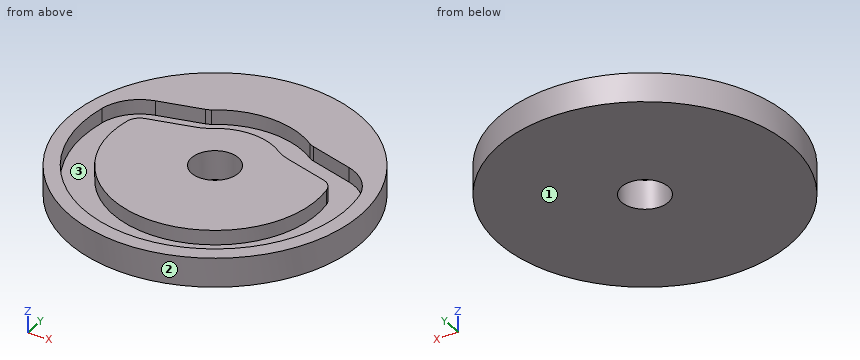
```python
from build123d import *

# Parameters (mm, degrees)
SKETCH_1_R            = 50
EXTRUDE_1_DEPTH       = 10
CUT_EXTRUDE_1_DEPTH   = 5
SKETCH_4_R            = 8
CUT_EXTRUDE_1_2_DEPTH = 72.414284285


with BuildPart() as part:
    # 草图1 → 凸台-拉伸1 (new body)
    with BuildSketch(Plane.XY):
        Circle(SKETCH_1_R)
    extrude(amount=EXTRUDE_1_DEPTH)

    # 草图2 → Cut-Extrude 1 (cut)
    with BuildSketch(Plane.XY.offset(10)):
        with BuildLine():
            ThreePointArc((44.226450487, 8.307892471), (0, -45), (-44.226450487, 8.307892471))
            ThreePointArc((-44.226450487, 8.307892471), (-40.486781839, 15.733956697), (-33.366586001, 20.027482375))
            Line((-33.366586001, 20.027482375), (-18.55842138, 23.995318126))
            ThreePointArc((-18.55842138, 23.995318126), (-17.756990045, 24.285259115), (-17.016442805, 24.70709765))
            ThreePointArc((-17.016442805, 24.70709765), (0, 30), (17.016442805, 24.70709765))
            ThreePointArc((17.016442805, 24.70709765), (17.756990045, 24.285259115), (18.55842138, 23.995318126))
            Line((18.55842138, 23.995318126), (33.366586001, 20.027482375))
            ThreePointArc((33.366586001, 20.027482375), (40.486781839, 15.733956697), (44.226450487, 8.307892471))
        make_face()
        with BuildLine():
            ThreePointArc((34.398350379, 6.461694144), (0, -35), (-34.398350379, 6.461694144))
            ThreePointArc((-34.398350379, 6.461694144), (-33.151794163, 8.937048886), (-30.77839555, 10.368224112))
            Line((-30.77839555, 10.368224112), (-15.970230929, 14.336059864))
            ThreePointArc((-15.970230929, 14.336059864), (-13.565936922, 15.20588283), (-11.344295203, 16.471398433))
            ThreePointArc((-11.344295203, 16.471398433), (0, 20), (11.344295203, 16.471398433))
            ThreePointArc((11.344295203, 16.471398433), (13.565936922, 15.20588283), (15.970230929, 14.336059864))
            Line((15.970230929, 14.336059864), (30.77839555, 10.368224112))
            ThreePointArc((30.77839555, 10.368224112), (33.151794163, 8.937048886), (34.398350379, 6.461694144))
        make_face(mode=Mode.SUBTRACT)
    extrude(amount=-CUT_EXTRUDE_1_DEPTH, mode=Mode.SUBTRACT)

    # 草图4 → Cut-Extrude 1 2 (cut, through all)
    with BuildSketch(Plane.XY.offset(10)):
        Circle(SKETCH_4_R)
    extrude(amount=-CUT_EXTRUDE_1_2_DEPTH, mode=Mode.SUBTRACT)


solid = part.part
```
Build history of the part. All positions in model axes, mm. Face numbers are marked on the shaded views. Round coordinates to 2 decimals unless told otherwise and drop trailing zeros. Write each loop counter-clockwise with the first axis right and the second up, starting at its lowest first coordinate (ties: lowest second). Pieces come first, ordered by that corner, then holes. Notation, with made-up numbers: (13.5, -4.5) -> (26.5, -4.5) arc R20 cw to (26.5, 7.5) -> close; hole circle Ø6 at (-6.75, -22). An arc over 180 degrees is marked (long way). Put each result on its own line as item: value.
Item 1: Wall check: probe 1 along Y at (x, z) = (-0.5, 8.75); probe 2 along Y at (x, z) = (19, 6); probe 3 along X at (y, z) = (-9, 6). Give the ranges that are in metal, low to high. Write a range as from..to.
Here are the results:
probe 1: y = -50..-45, -35..-7.98, 7.98..19.99, 30..50
probe 2: y = -46.25..-40.79, -29.39..13.52, 23.88..46.25
probe 3: x = -49.18..-44.09, -33.82..33.82, 44.09..49.18
Item 2: Two-plate mould, pull along Y, no slides. Class the marked faces 1, 2 and 3: pulls with the +Y half, pulls with the -Y half, needs draft (parallel to the pull), parting line crosses it, or undercut.
Here are the results:
face 1: needs draft
face 2: parting line crosses it
face 3: undercut
Item 3: Slice it at B-B, the plane x = 0. Give the cut face in (y, z), plus the area to 3 significant figures.
Here are the results:
outline: (-50, 0) -> (-8, 0) -> (-8, 10) -> (-35, 10) -> (-35, 5) -> (-45, 5) -> (-45, 10) -> (-50, 10) -> close; (8, 0) -> (50, 0) -> (50, 10) -> (30, 10) -> (30, 5) -> (20, 5) -> (20, 10) -> (8, 10) -> close
area: 740 mm^2
Item 4: Slice it at A-A, the plane z = 7.5. Give the cut face in (x, y), plus the area to 3 significant figures.
Here are the results:
outline: circle Ø100 at (0, 0); (-34.4, 6.46) arc R35 ccw (long way) to (34.4, 6.46) arc R5 ccw to (30.78, 10.37) -> (15.97, 14.34) arc R15 cw to (11.34, 16.47) arc R20 ccw to (-11.34, 16.47) arc R15 cw to (-15.97, 14.34) -> (-30.78, 10.37) arc R5 ccw to start; hole (-44.23, 8.31) arc R45 ccw (long way) to (44.23, 8.31) arc R15 ccw to (33.37, 20.03) -> (18.56, 24) arc R5 cw to (17.02, 24.71) arc R30 ccw to (-17.02, 24.71) arc R5 cw to (-18.56, 24) -> (-33.37, 20.03) arc R15 ccw to start; hole circle Ø16 at (0, 0)
area: 5,350 mm^2
Item 5: Slice it at D-D, the plane z = 1.25. Give the cut face in (x, y).
Here are the results:
outline: circle Ø100 at (0, 0); hole circle Ø16 at (0, 0)
Item 6: Slice it at C-C, the plane y = 0. Give the cut face in (x, z).
Here are the results:
outline: (-50, 0) -> (-8, 0) -> (-8, 10) -> (-35, 10) -> (-35, 5) -> (-45, 5) -> (-45, 10) -> (-50, 10) -> close; (8, 0) -> (50, 0) -> (50, 10) -> (45, 10) -> (45, 5) -> (35, 5) -> (35, 10) -> (8, 10) -> close
Item 7: Flat gauge pins, fed straight in: P1, Ø2, axis at y = -24, z = 6, coming from the -X side; P2, Ø6, axis at y = -15.5, z = 4, coming from the -X side; P3, Ø6, axis at x = 27, y = -24, coming from the -Z side; P4, Ø1, axis at y = -37, z = 3, coming from the -X side. Where does each tip first touch, or does it go through?
Here are the results:
P1: stops at x = -44.4
P2: stops at x = -48.41
P3: stops at z = 0
P4: stops at x = -34.17
